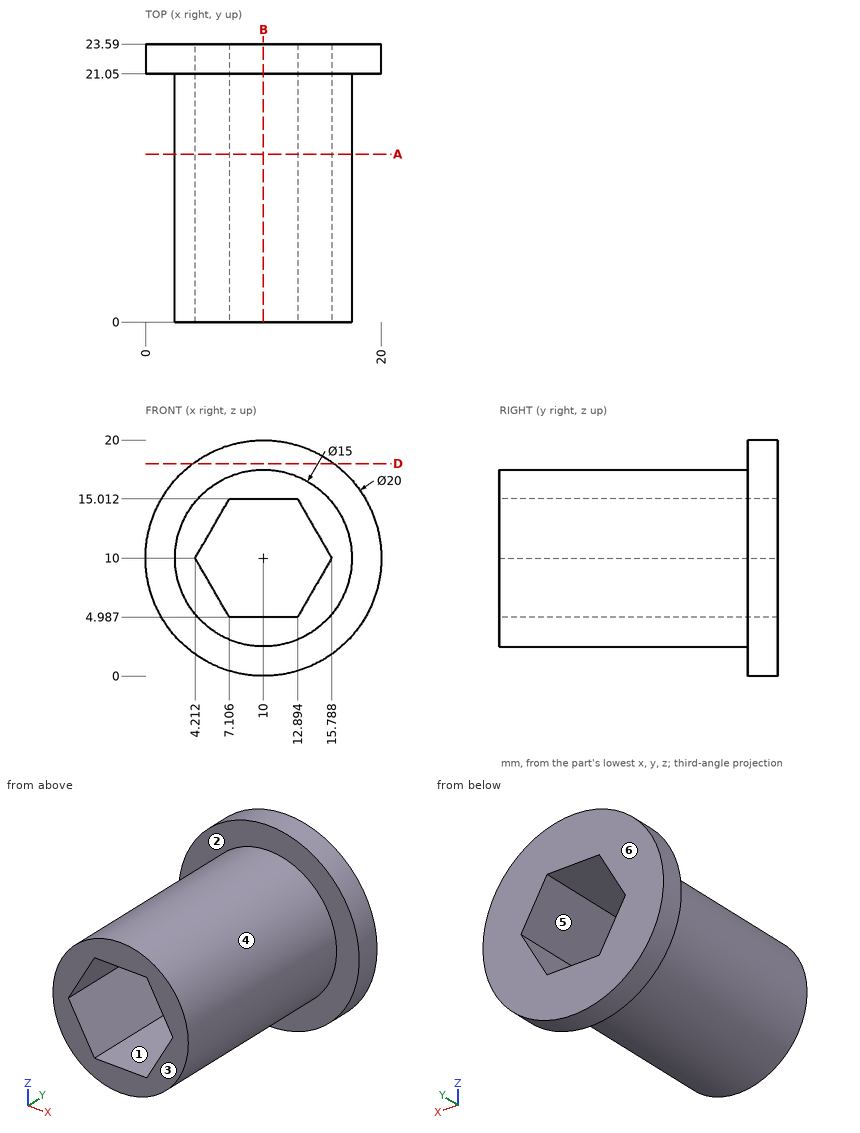
For this review, use the dimensioned drawing (mm, ordinates from the lowest corner) and the shaded views. A direction names the side the tool comes from. Give positions to 0.01 mm unless a question says otherwise; leave off trailing zeros. Loops run counter-clockwise (first coordinate to the right, second up) from the corner with the lowest first, then second, coordinate; pieces in that order, holes last.
Item 1: Draft analysis for pull direction X (two halves, no side actions). For the marked faces 4, 5 and 6, state which applies: +X half, -X half, draft (parallel to the pull), parting line (faces both ways), or undercut.
Item 2: Take a section at A-A, the plane y = 14.25. State the section outline as (x, z) points.
Item 3: Take a section at D-D, the plane z = 18. State the section outline as (x, y) points.
Item 4: Tool access review of the marked faces 1, 2 and 3: name each direction out of +Z, -Z, +X, -X, +Y, -Y from which nothing blocks a thin tool from reaching the whole face with its end or side.
Item 5: For line 1 along Z through (x, y) = (9.75, 18.25) (1 decimal); line 2 along Y through (x, z) = (13.25, 18); line 3 along X through (y, z) = (9, 11) (1 decimal), list the stretches that pass through material, from the lowest coordinate up.
Item 6: Insertion check: pin 1 (1 mm diameter, centred on y = 16, z = 15.5, fed in from -X); pin 2 (1.5 mm diameter, centred on y = 20, z = 5.5, fed in from -X) (1 decimal); pin 3 (1 mm diameter, centred on x = 14, y = 11.5, fed in from +Z). Each pin has a flat end and moves straight along its axis. Give the tip position at first contact, or say it passes through.
Item 7: Take a section at B-B, the plane x = 10. State the section outline as (y, z) points, and give its area (3 significant figures).
Calculated:
1. face 4: parting line
1. face 5: undercut
1. face 6: draft
2. outline: circle Ø15 at (10, 10); hole (4.21, 10) - (7.11, 4.99) - (12.89, 4.99) - (15.79, 10) - (12.89, 15.01) - (7.11, 15.01) - close
3. outline: (4, 21.05) - (16, 21.05) - (16, 23.59) - (4, 23.59) - close
4. face 1: +Y, -Y
4. face 2: -Y
4. face 3: +Z, -Z, +X, -X, -Y
5. line 1: z = 2.5 to 5, 15 to 17.5
5. line 2: y = 21.05 to 23.59
5. line 3: x = 2.6 to 4.8, 15.2 to 17.4
6. pin 1: stops at x = 4.41
6. pin 2: stops at x = 3.5
6. pin 3: stops at z = 16.63
7. outline: (0, 2.5) - (21.05, 2.5) - (21.05, 0) - (23.59, 0) - (23.59, 4.99) - (0, 4.99) - close; (0, 15.01) - (23.59, 15.01) - (23.59, 20) - (21.05, 20) - (21.05, 17.5) - (0, 17.5) - close
7. area: 130 mm2
